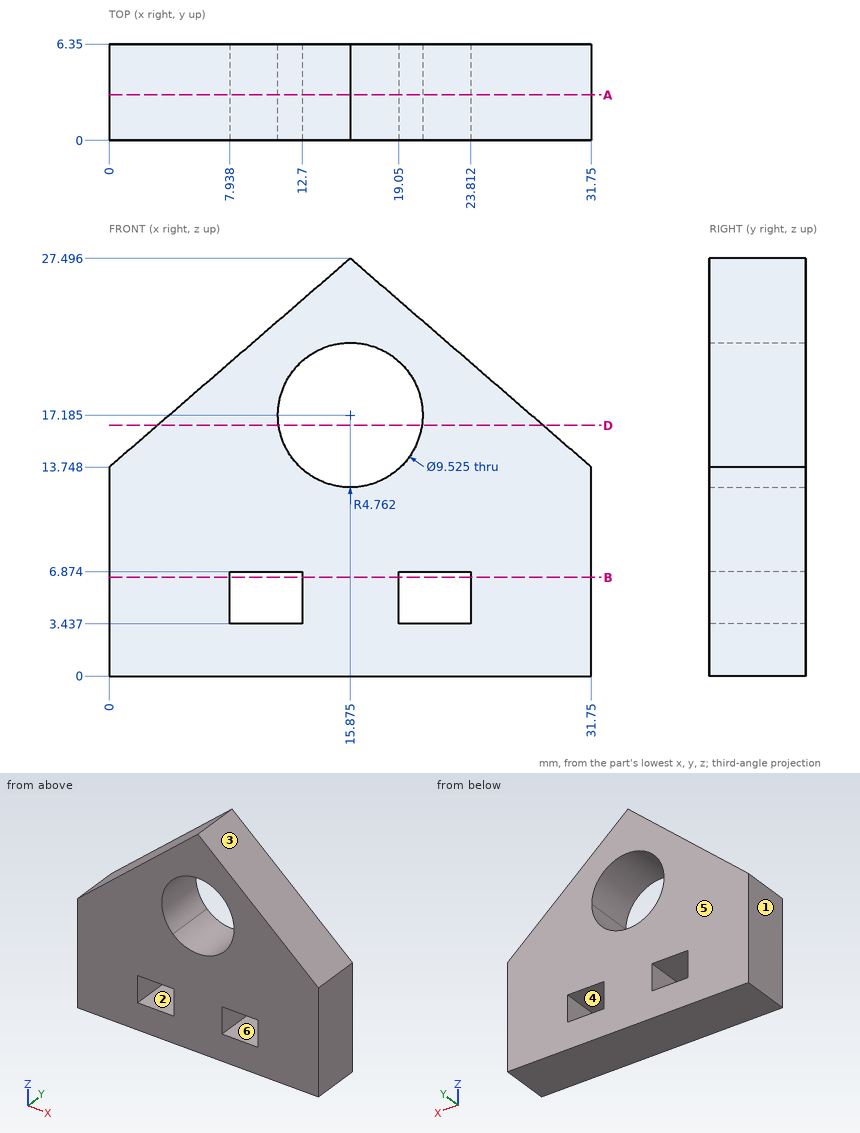
Print and shaded views of the part. All mm, measured from the part's lowest x, y and z. A direction names the side the tool comes from. Round coordinates to 2 decimals unless told otherwise and drop trailing zeros. Write each loop counter-clockwise with the first axis right and the second up, starting at its lowest first coordinate (ties: lowest second). Pieces come first, ordered by that corner, then holes.
(1) Slice it at A-A, the plane y = 3. Count the separate pieces of the cut face and the enclosed holes in it, and give its area (3 significant figures).
(2) Slice it at D-D, the plane z = 16.5. Write the cut outline in (x, y), and give its area (3 significant figures).
(3) Probe line 1 along X through (y, z) = (2.5, 6.75); line 2 along Z through (x, y) = (11.5, 3.5) (1 decimal); line 3 along X through (y, z) = (1.75, 20.5) (1 decimal). List the from-to ranges inside material, lowest first.
(4) Slice it at B-B, the plane z = 6.5. Write the cut outline in (x, y).
(5) Mould opens along Z. For the marked faces 1, 2, 3 and 4 say: pulls with the +Z half, pulls with the -Z half, needs draft (parallel to the pull), parting line crosses it, or undercut.
(6) Drop flat-ended pins along their axis: P1, Ø1.5, axis at y = 1.5, z = 23.5, coming from the -X side (1 decimal); P2, Ø1, axis at x = 6.5, y = 1.5, coming from the +Z side. Give the stop position or say it passes through.
(7) 3-axis set-ups, long thin cutter, end or side, ignore diameter. For the marked faces 5 and 6: which of +Z, -Z, +X, -X, +Y, -Y reach the whole face in a straight line?
From the geometry:
1. separate pieces: 1
1. enclosed holes: 3
1. area: 551 mm2
2. outline: (3.18, 0) - (11.16, 0) - (11.16, 6.35) - (3.18, 6.35) - close; (20.59, 0) - (28.57, 0) - (28.57, 6.35) - (20.59, 6.35) - close
2. area: 101 mm2
3. line 1: x = 0 to 7.94, 12.7 to 19.05, 23.81 to 31.75
3. line 2: z = 0 to 3.4, 6.9 to 15.3, 19.1 to 23.7
3. line 3: x = 7.8 to 12.5, 19.3 to 24
4. outline: (0, 0) - (7.94, 0) - (7.94, 6.35) - (0, 6.35) - close; (12.7, 0) - (19.05, 0) - (19.05, 6.35) - (12.7, 6.35) - close; (23.81, 0) - (31.75, 0) - (31.75, 6.35) - (23.81, 6.35) - close
5. face 1: needs draft
5. face 2: undercut
5. face 3: pulls with the +Z half
5. face 4: undercut
6. P1: stops at x = 10.4
6. P2: stops at z = 19.81
7. face 5: +Z, -Z, +X, -X, +Y
7. face 6: +Y, -Y
